For this review, take the finished solid that the model builds, in its own axes (mm). Face numbers are marked on the shaded views. Give positions to 0.01 mm unless a question says otherwise; leave off trailing zeros. Loops run counter-clockwise (first coordinate to the right, second up) from the corner with the lowest first, then second, coordinate; pieces in that order, holes last.
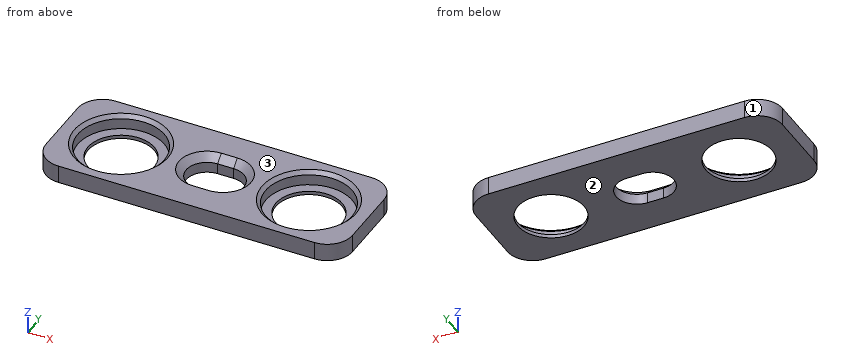
```python
from build123d import *

# Parameters (mm, degrees)
CROQUIS1_W              = 85.583933156
CROQUIS1_H              = 31.172413686
CROQUIS1_R              = 12.075
SALIENTE_EXTRUIR1_DEPTH = 5
CROQUIS2_W              = 85.583933156
CROQUIS2_H              = 31.172413686
CROQUIS2_R              = 9.25
SALIENTE_EXTRUIR2_DEPTH = 1
REDONDEO1_R             = 7
CORTAR_EXTRUIR1_DEPTH   = 46.815742353
CHAFL_N1_SIZE           = 2
CHAFL_N2_SIZE           = 1


with BuildPart() as part:
    # Croquis1 → Saliente-Extruir1 (new body)
    with BuildSketch(Plane.XY):
        Rectangle(CROQUIS1_W, CROQUIS1_H)
        with Locations((-26.25, 0)):
            Circle(CROQUIS1_R, mode=Mode.SUBTRACT)
        with Locations((26.25, 0)):
            Circle(CROQUIS1_R, mode=Mode.SUBTRACT)
    extrude(amount=SALIENTE_EXTRUIR1_DEPTH)

    # Croquis2 → Saliente-Extruir2 (add)
    with BuildSketch(Plane(origin=(0, 0, 0), x_dir=(-1, 0, 0), z_dir=(0, 0, -1))):
        Rectangle(CROQUIS2_W, CROQUIS2_H)
        with Locations((-26.25, 0)):
            Circle(CROQUIS2_R, mode=Mode.SUBTRACT)
        with Locations((26.25, 0)):
            Circle(CROQUIS2_R, mode=Mode.SUBTRACT)
    extrude(amount=-SALIENTE_EXTRUIR2_DEPTH)

    # Redondeo1
    redondeo1_edges = [part.edges().sort_by_distance(p)[0] for p in [
        (42.791966578, -15.586206843, 2.5),
        (-42.791966578, -15.586206843, 2.5),
        (-42.791966578, 15.586206843, 2.5),
        (42.791966578, 15.586206843, 2.5),
    ]]
    fillet(redondeo1_edges, radius=REDONDEO1_R)

    # Croquis3 → Cortar-Extruir1 (cut, through all)
    with BuildSketch(Plane.XY.offset(5)):
        with BuildLine():
            Line((-2.24145708, 5.808706223), (2.24145708, 5.808706223))
            ThreePointArc((2.24145708, 5.808706223), (8.050163302, 0), (2.24145708, -5.808706223))
            Line((2.24145708, -5.808706223), (-2.24145708, -5.808706223))
            ThreePointArc((-2.24145708, -5.808706223), (-8.050163302, 0), (-2.24145708, 5.808706223))
        make_face()
    extrude(amount=-CORTAR_EXTRUIR1_DEPTH, mode=Mode.SUBTRACT)

    # Chaflán1
    chafl_n1_edges = [part.edges().sort_by_distance(p)[0] for p in [
        (-8.050163302, 0, 5),
        (0, -5.808706223, 5),
        (8.050163302, 0, 5),
        (0, 5.808706223, 5),
    ]]
    chamfer(chafl_n1_edges, length=CHAFL_N1_SIZE)

    # Chaflán2
    chafl_n2_edges = [part.edges().sort_by_distance(p)[0] for p in [
        (-38.325, 0, 5),
        (14.175, 0, 5),
    ]]
    chamfer(chafl_n2_edges, length=CHAFL_N2_SIZE)


solid = part.part
```
Q1. For pin 1 Ø12 at (x, y) = (25, 2.5) entering from +Z; pin 2 Ø1 at (x, y) = (-20.5, -8.5) entering from +Z, all flat-tipped, find the tip position at first contact; note any pin that passes through.
Answers:
pin 1: passes through
pin 2: stops at z = 1
Q2. Consider section C-C on z = 1.95. Give the boundary of the cut face in (x, y) (3 decimals), plus the area to 3 significant figures.
Answers:
outline: (-42.792, -8.586) arc R7 ccw to (-35.792, -15.586) - (35.792, -15.586) arc R7 ccw to (42.792, -8.586) - (42.792, 8.586) arc R7 ccw to (35.792, 15.586) - (-35.792, 15.586) arc R7 ccw to (-42.792, 8.586) - close; hole circle Ø24.15 at (-26.25, 0); hole (-2.241, -5.809) - (2.241, -5.809) arc R5.809 ccw to (2.241, 5.809) - (-2.241, 5.809) arc R5.809 ccw to start; hole circle Ø24.15 at (26.25, 0)
area: 1,550 mm2
Q3. Mouldability with a two-part tool opening along Z and no side actions: class the marked faces 1, 2 and 3 as +Z half, -Z half, draft (parallel to the pull), parting line (faces both ways), or undercut.
Answers:
face 1: draft
face 2: -Z half
face 3: +Z half
Q4. Consider section B-B on y = 0. Count the separate pieces of the cut face and the enclosed holes in it, plus the area to 3 significant figures.
Answers:
separate pieces: 4
enclosed holes: 0
area: 111 mm2
Q5. For probe 1 along X at (y, z) = (0, 2.1) (3 decimals); probe 2 along X at (y, z) = (-6, 1.4); probe 3 along X at (y, z) = (8.5, 1.35), list the stretches that pass through material, from the lowest coordinate up.
Answers:
probe 1: x = -42.792 to -38.325, -14.175 to -8.05, 8.05 to 14.175, 38.325 to 42.792
probe 2: x = -42.79 to -36.73, -15.77 to 15.77, 36.73 to 42.79
probe 3: x = -42.79 to -34.83, -17.67 to 17.67, 34.83 to 42.79
Q6. Consider section A-A on x = -26.25. Give the boundary of the cut face in (y, z) (3 decimals).
Answers:
outline: (-15.586, 0) - (-9.25, 0) - (-9.25, 1) - (-12.075, 1) - (-12.075, 4) - (-13.075, 5) - (-15.586, 5) - close; (9.25, 0) - (15.586, 0) - (15.586, 5) - (13.075, 5) - (12.075, 4) - (12.075, 1) - (9.25, 1) - close
